The drawing under review shows one solid part. Ordinate dimensions are in mm from its lowest x, y, z. Round coordinates to 2 decimals unless told otherwise and drop trailing zeros. Order: outer loops, then holes, each group sorted by start corner. A loop starts at its lowest first (then second) coordinate and runs counter-clockwise, first axis right, second up. Notation, with made-up numbers: M 31,0 L 76,0 A30 cw 76,37 Z; hole C -24,21 d3. An arc over 180 degrees is marked long. Answer as a JSON object with one key per item and string values. Group by question number.
1. Add section D-D on y = 29. State the section outline as (x, z) points.
2. To check wall thickness, follow probe 1 along X at (y, z) = (25.5, 16.5). State the ranges of the line that lie inside material, in increasing order. Write a range as [from, to].
3. Clearance check with flat-ended pins moving along their axes: P1, Ø1.5, axis at x = 36.5, z = 10.5, coming from the +Y side; P2, Ø1.5, axis at y = 42.5, z = 12, coming from the -X side; P3, Ø4.5, axis at x = 18.24, z = 33.75, coming from the +Y side; P4, Ø0.6, axis at x = 0.5, z = 26, coming from the -Y side. State where each tip first meets the part, or that it passes through.
4. Mouldability with a two-part tool opening along X and no side actions: class the marked faces 1, 2 and 3 as released by +X, released by -X, zero draft, split by the parting line, or undercut.
5. Add section B-B on z = 22.5. State the section outline as (x, y) points (1 decimal).
6. Add section C-C on z = 38. State the section outline as (x, y) points.
7. Add section A-A on x = 5.5. State the section outline as (y, z) points.
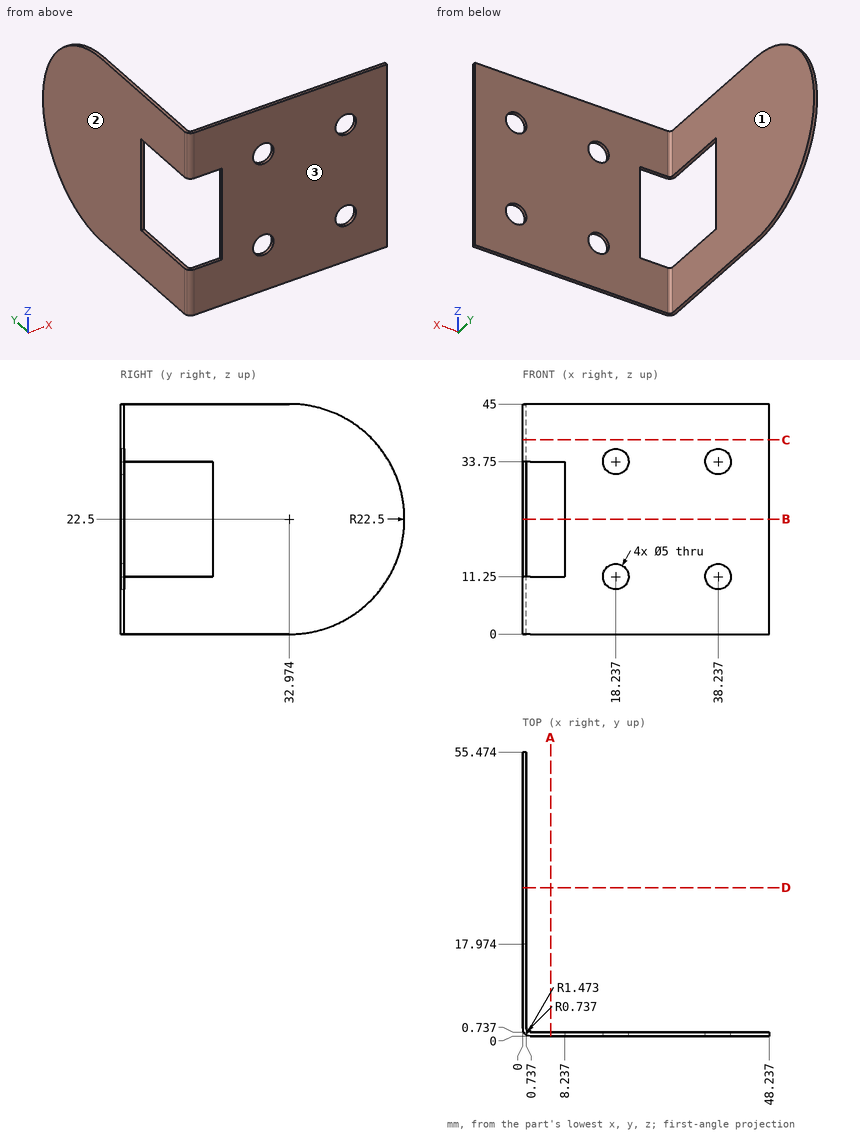
Recorded:
{
 "1": {"outline": "M 0,0 L 0.74,0 L 0.74,45 L 0,45 Z"},
 "2": {"probe 1": "x = [0, 0.74]"},
 "3": {"P1": "stops at y = 0.74", "P2": "stops at x = 0", "P3": "passes through", "P4": "stops at y = 17.97"},
 "4": {"face 1": "released by +X", "face 2": "released by -X", "face 3": "zero draft"},
 "5": {"outline": "M 0,18 L 0.7,18 L 0.7,55.5 L 0,55.5 Z; M 8.2,0 L 48.2,0 L 48.2,0.7 L 8.2,0.7 Z"},
 "6": {"outline": "M 0,1.47 A1.47 ccw 1.47,0 L 48.24,0 L 48.24,0.74 L 1.47,0.74 A0.74 cw 0.74,1.47 L 0.74,49.28 L 0,49.28 Z"},
 "7": {"outline": "M 0,0 L 0.74,0 L 0.74,11.25 L 0,11.25 Z; M 0,33.75 L 0.74,33.75 L 0.74,45 L 0,45 Z"}
}
